from build123d import *

# Parameters (mm, degrees)
BOSS_EXTRUDE1_DEPTH = 3


with BuildPart() as part:
    # Sketch1 → Boss-Extrude1 (new body)
    with BuildSketch(Plane(origin=(0, 0, 0), x_dir=(1, 0, 0), z_dir=(0, 1, 0))):
        with BuildLine():
            ThreePointArc((-44.190268387, -41.389735818), (-39.823508359, -45.131010371), (-34.090908396, -44.680426216))
            ThreePointArc((-34.090908396, -44.680426216), (-7.1e-08, -36.484692283), (34.090908269, -44.680426152))
            ThreePointArc((34.090908269, -44.680426152), (39.823508354, -45.131010372), (44.190268446, -41.389735701))
            ThreePointArc((44.190268446, -41.389735701), (49.538672672, -18.999999828), (44.19026829, 3.389736008))
            ThreePointArc((44.19026829, 3.389736008), (42.526729152, 5.566147144), (40.192590574, 6.999996857))
            ThreePointArc((40.192590574, 6.999996857), (22.010436955, 18.032282207), (8.819043592, 34.714283628))
            ThreePointArc((8.819043592, 34.714283628), (7.4e-08, 40), (-8.819043522, 34.714283759))
            ThreePointArc((-8.819043522, 34.714283759), (-22.010436745, 18.032282393), (-40.19259019, 6.999997005))
            ThreePointArc((-40.19259019, 6.999997005), (-42.526728969, 5.566147309), (-44.190268254, 3.389736081))
            ThreePointArc((-44.190268254, 3.389736081), (-49.538672672, -18.999999853), (-44.190268387, -41.389735818))
        make_face()
    extrude(amount=BOSS_EXTRUDE1_DEPTH)


solid = part.part
Source: CAD feature listing. Evaluate the final solid. Frame: model axes, mm. Round coordinates to 2 decimals unless told otherwise and drop trailing zeros. Loops run counter-clockwise (first coordinate to the right, second up) from the corner with the lowest first, then second, coordinate; pieces in that order, holes last. Notation, with made-up numbers: M 13.5,-7 L 49.5,-7 A15 ccw 49.5,-2 Z; hole C -28.75,-9.75 d2. An arc over 180 degrees is marked long. Return JSON: item names as keys, results as strings. Group by question number.
1. Section query C-C on z = -20.5. Output: boundary loops of the cut face in (x, y).
2. Mould query, pull axis X, two halves, no side actions, for faces 1 (the face through (22.24, 1.48, -17.83)), 2 (the face through (-39.902, 1.479, 45.105)), 3 (the face through (-1, 3, 12)). Classes: released by +X, released by -X, zero draft, split by the parting line, or undercut.
3. Section query B-B on x = -42. Output: boundary loops of the cut face in (y, z).
4. Pin query (flat end, axial travel): pin 1 (1.5 mm diameter, centred on y = 1, z = 8, fed in from +X). Return the tip coordinate at first contact, or that it passes through.
5. Section query A-A on y = 1.75. Output: boundary loops of the cut face in (x, z), and give its area (3 significant figures).
6. Material intervals for line 1 along X through (y, z) = (0.85, 42); line 2 along Z through (x, y) = (-4, 2.5); line 3 along Z through (x, y) = (7, 0.6), sorted ascending. Write a range as from..to.
Checks:
{
 "1": {"outline": "M -19.38,0 L 19.38,0 L 19.38,3 L -19.38,3 Z"},
 "2": {"face 1": "released by +X", "face 2": "undercut", "face 3": "zero draft"},
 "3": {"outline": "M 0,-6 L 3,-6 L 3,44 L 0,44 Z"},
 "4": {"pin 1": "stops at x = 48.47"},
 "5": {"outline": "M -44.19,-3.39 A7.5 ccw -40.19,-7 A60 cw -8.82,-34.71 A10 ccw 8.82,-34.71 A60 cw 40.19,-7 A7.5 ccw 44.19,-3.39 A49.54 ccw 44.19,41.39 A7.5 ccw 34.09,44.68 A75 cw -34.09,44.68 A7.5 ccw -44.19,41.39 A49.54 ccw Z", "area": "5,710 mm²"},
 "6": {"line 1": "x = -43.84..-28.23, 28.23..43.84", "line 2": "z = -39.17..36.59", "line 3": "z = -37.14..36.81"}
}
